from build123d import *

# Parameters (mm, degrees)
EXTRUDE_THIN1_DEPTH = 349.25
FILLET1_R           = 1.27


with BuildPart() as part:
    # Sketch1 → Extrude-Thin1 (new body)
    with BuildSketch(Plane.XY):
        with BuildLine():
            Line((0, 34.925), (-15.08125, 34.925))
            Line((-15.08125, 34.925), (-15.08125, 22.225))
            Line((-15.08125, 22.225), (-12.589163559, 22.225))
            ThreePointArc((-12.589163559, 22.225), (-12.244128802, 16.434292536), (-9.935478518, 11.1125))
            ThreePointArc((-9.935478518, 11.1125), (-7.626828235, 5.790707464), (-7.281793478, 0))
            Line((-7.281793478, 0), (-3.313043478, 0))
            Line((-3.313043478, 0), (-3.313043478, 1.27))
            Line((-3.313043478, 1.27), (-5.912702406, 1.27))
            ThreePointArc((-5.912702406, 1.27), (-6.570184472, 6.773148448), (-8.876108727, 11.812953884))
            ThreePointArc((-8.876108727, 11.812953884), (-11.159248724, 17.431038769), (-11.096159817, 23.495))
            Line((-11.096159817, 23.495), (-13.81125, 23.495))
            Line((-13.81125, 23.495), (-13.81125, 33.655))
            Line((-13.81125, 33.655), (0, 33.655))
            Line((0, 33.655), (0, 34.925))
        make_face()
    extrude(amount=-EXTRUDE_THIN1_DEPTH)

    # Fillet1
    fillet1_edges = [part.edges().sort_by_distance(p)[0] for p in [
        (-7.281793478, 0, -174.625),
        (-15.08125, 22.225, -174.625),
        (-15.08125, 34.925, -174.625),
        (-11.096159817, 23.495, -174.625),
    ]]
    fillet(fillet1_edges, radius=FILLET1_R)


solid = part.part
Could you check a few things on this model? Use its own coordinates, in mm. A direction names the side the tool comes from. Round coordinates to 2 decimals unless told otherwise and drop trailing zeros. Order: outer loops, then holes, each group sorted by start corner. A loop starts at its lowest first (then second) coordinate and runs counter-clockwise, first axis right, second up.
(1) Imagine slicing it at B-B (y = 5). Write out the boundary of the cut face in (x, z).
Response values:
outline: (-7.46, -349.25) - (-6.17, -349.25) - (-6.17, 0) - (-7.46, 0) - close
(2) If we mould it in two halves opening along Y, with no side actions, what happens to faces 1 (the flat face through (-15.081, 29, -172)), 2 (the cylindrical face through (-11, 16.7, -172.2)), 3 (the flat face through (-7, 34.925, -172))? For each: released by +Y, released by -Y, zero draft, split by the parting line, or undercut.
Response values:
face 1: zero draft
face 2: undercut
face 3: released by +Y
(3) Imagine slicing it at A-A (z = -86.5). Write out the boundary of the cut face in (x, y) (1 decimal).
Response values:
outline: (-15.1, 23.5) arc R1.3 ccw to (-13.8, 22.2) - (-12.6, 22.2) arc R16.7 ccw to (-9.9, 11.1) arc R16.7 cw to (-7.2, 1.3) arc R1.3 ccw to (-5.9, 0) - (-3.3, 0) - (-3.3, 1.3) - (-5.9, 1.3) arc R17.9 ccw to (-8.9, 11.8) arc R15.4 cw to (-11.3, 22.1) arc R1.3 ccw to (-12.6, 23.5) - (-13.8, 23.5) - (-13.8, 33.7) - (0, 33.7) - (0, 34.9) - (-13.8, 34.9) arc R1.3 ccw to (-15.1, 33.7) - close
(4) I'm going to push flat-ended pins straight in: pin 1 (1 mm diameter, centred on y = 0.5, z = -137, fed in from +X); pin 2 (1.5 mm diameter, centred on y = 13.5, z = -149.5, fed in from -X); pin 3 (2 mm diameter, centred on x = -13, y = 11, fed in from -Z); pin 4 (11 mm diameter, centred on y = 26.5, z = -197.5, fed in from +X). Where does each tip first touch, or does it pass through?
Response values:
pin 1: stops at x = -3.31
pin 2: stops at x = -11.56
pin 3: passes through
pin 4: stops at x = -11.32
(5) Which directions (+Z, -Z, +X, -X, +Y, -Y) give clear straight access to the entire face, cutting with the end or side of a thin tool? Please do faces 4 (the cylindrical face through (-6.55, 6.7, -172.18)), 5 (the flat face through (-12, 21, -349.25)).
Response values:
face 4: +Z, -Z, +X
face 5: -Z, +X, -X, +Y, -Y
(6) Imagine slicing it at C-C (y = 18.5). Write out the boundary of the cut face in (x, z).
Response values:
outline: (-12.6, -349.25) - (-11.32, -349.25) - (-11.32, 0) - (-12.6, 0) - close
(7) Please list where these lines run through material, in increasing order: line 1 along Y through (x, z) = (-13.5, -235) (3 decimals); line 2 along Y through (x, z) = (-4, -251) (3 decimals); line 3 along X through (y, z) = (19.5, -237).
Response values:
line 1: y = 22.225 to 23.495, 33.655 to 34.925
line 2: y = 0 to 1.27, 33.655 to 34.925
line 3: x = -12.68 to -11.41
